The model under review builds one solid part; all positions refer to its coordinate system, in mm. Round coordinates to 2 decimals unless told otherwise and drop trailing zeros. Order: outer loops, then holes, each group sorted by start corner. A loop starts at its lowest first (then second) coordinate and runs counter-clockwise, first axis right, second up. Notation, with made-up numbers: (78.5, 89) -> (121.5, 89) arc R16 ccw to (121.5, 94) -> close; hole circle Ø10 at (-23.75, 55.5). An arc over 180 degrees is marked (long way). Return JSON: item names as keys, results as strings. Group by question number.
from build123d import *

# Parameters (mm, degrees)
SKETCH_1_R           = 45
SKETCH_1_R_2         = 1.65
SKETCH_1_R_3         = 10.15
EXTRUDE_1_DEPTH      = 10
SKETCH_2_R           = 4.05
CUT_EXTRUDE_1_DEPTH  = 12
SKETCH_5_R           = 34.5
CUT_EXTRUDE_4_DEPTH  = 3
CUT_EXTRUDE_6_DEPTH  = 3
SKETCH_10_R          = 45
CUT_EXTRUDE_9_DEPTH  = 8
SKETCH_11_R          = 11.25
CUT_EXTRUDE_10_DEPTH = 10


with BuildPart() as part:
    # 草图1 → 凸台-拉伸1 (new body)
    with BuildSketch(Plane.XY):
        Circle(SKETCH_1_R)
        with Locations((-28.991378029, 28.991378029)):
            Circle(SKETCH_1_R_2, mode=Mode.SUBTRACT)
        with Locations((28.991378029, 28.991378029)):
            Circle(SKETCH_1_R_2, mode=Mode.SUBTRACT)
        with Locations((-28.991378029, -28.991378029)):
            Circle(SKETCH_1_R_2, mode=Mode.SUBTRACT)
        with Locations((28.991378029, -28.991378029)):
            Circle(SKETCH_1_R_2, mode=Mode.SUBTRACT)
        with Locations((0, 29)):
            Circle(SKETCH_1_R_2, mode=Mode.SUBTRACT)
        with Locations((-25.11473671, -14.5)):
            Circle(SKETCH_1_R_2, mode=Mode.SUBTRACT)
        with Locations((25.11473671, -14.5)):
            Circle(SKETCH_1_R_2, mode=Mode.SUBTRACT)
        Circle(SKETCH_1_R_3, mode=Mode.SUBTRACT)
    extrude(amount=EXTRUDE_1_DEPTH)

    # 草图2 → 切除-拉伸1 (cut)
    with BuildSketch(Plane.XY.offset(10)):
        with Locations((0, 19.25)):
            Circle(SKETCH_2_R)
    extrude(amount=-CUT_EXTRUDE_1_DEPTH, mode=Mode.SUBTRACT)

    # 草图5 → 切除-拉伸4 (cut)
    with BuildSketch(Plane(origin=(0, 0, 0), x_dir=(-1, 0, 0), z_dir=(0, 0, -1))):
        Circle(SKETCH_5_R)
    extrude(amount=-CUT_EXTRUDE_4_DEPTH, mode=Mode.SUBTRACT)

    # 草图7 → 切除-拉伸6 (cut)
    with BuildSketch(Plane(origin=(0, 0, 3), x_dir=(-1, 0, 0), z_dir=(0, 0, -1))):
        Polygon((0, 0), (-25.071115349, -53.76518037), (25.215961405, -54.075803739), align=None)
    extrude(amount=CUT_EXTRUDE_6_DEPTH, mode=Mode.SUBTRACT)

    # 草图10 → 切除-拉伸9 (cut)
    with BuildSketch(Plane(origin=(0, 0, 0), x_dir=(-1, 0, 0), z_dir=(0, 0, -1))):
        Circle(SKETCH_10_R)
    extrude(amount=-CUT_EXTRUDE_9_DEPTH, mode=Mode.SUBTRACT)

    # 草图11 → 切除-拉伸10 (cut)
    with BuildSketch(Plane(origin=(0, 0, 8), x_dir=(-1, 0, 0), z_dir=(0, 0, -1))):
        Circle(SKETCH_11_R)
    extrude(amount=-CUT_EXTRUDE_10_DEPTH, mode=Mode.SUBTRACT)


solid = part.part
Item 1: Wall thickness on line 1 along X through (y, z) = (0.5, 9.6); line 2 along X through (y, z) = (-13, 8.4); line 3 along Y through (x, z) = (3, 8.15): over which ranges is each line inside the solid? List them lowest first.
Item 2: Consider section C-C on x = 9.5. State the section outline as (y, z) points.
Item 3: Insertion check: pin 1 Ø1 at (x, z) = (-8, 9.5) entering from +Y. The pin has a flat end and moves straight along its axis. Give the tip position at first contact, or say it passes through.
Item 4: Consider section B-B on y = 0. State the section outline as (x, z) points, plus the area to 3 significant figures.
Item 5: Consider section D-D on y = -14.5. State the section outline as (x, z) points.
Item 6: The part is to be moulded in two halves that separate along X. For faces 1 (the face through (30.516, -29.623, 8.986)), 2 (the face through (9, -9, 10)), 3 (the face through (-5.19, -9.98, 8.99)), 4 (the face through (20.765, -39.923, 8.986)), say which applies: +X half, -X half, draft (parallel to the pull), parting line (faces both ways), or undercut.
Item 7: Consider section A-A on x = 0. State the section outline as (y, z) points, plus the area to 3 significant figures.
Values:
{
 "1": {"line 1": "-45 to -11.24, 11.24 to 45", "line 2": "-43.08 to -25.8, -24.43 to 24.43, 25.8 to 43.08", "line 3": "-44.9 to -10.84, 10.84 to 16.53, 21.97 to 44.9"},
 "2": {"outline": "(-43.99, 8) -> (-6.03, 8) -> (-6.03, 10) -> (-43.99, 10) -> close; (6.03, 8) -> (43.99, 8) -> (43.99, 10) -> (6.03, 10) -> close"},
 "3": {"pin 1": "y = 44.37"},
 "4": {"outline": "(-45, 8) -> (-11.25, 8) -> (-11.25, 10) -> (-45, 10) -> close; (11.25, 8) -> (45, 8) -> (45, 10) -> (11.25, 10) -> close", "area": "135 mm^2"},
 "5": {"outline": "(-42.6, 8) -> (-26.76, 8) -> (-26.76, 10) -> (-42.6, 10) -> close; (-23.46, 8) -> (23.46, 8) -> (23.46, 10) -> (-23.46, 10) -> close; (26.76, 8) -> (42.6, 8) -> (42.6, 10) -> (26.76, 10) -> close"},
 "6": {"face 1": "undercut", "face 2": "draft", "face 3": "undercut", "face 4": "parting line"},
 "7": {"outline": "(-45, 8) -> (-11.25, 8) -> (-11.25, 10) -> (-45, 10) -> close; (11.25, 8) -> (15.2, 8) -> (15.2, 10) -> (11.25, 10) -> close; (23.3, 8) -> (27.35, 8) -> (27.35, 10) -> (23.3, 10) -> close; (30.65, 8) -> (45, 8) -> (45, 10) -> (30.65, 10) -> close", "area": "112 mm^2"}
}
